```python
from build123d import *

# Parameters (mm, degrees)
SKETCH1_R               = 3.175
SKETCH1_R_2             = 4.025
BOSS_EXTRUDE1_DEPTH     = 6.35
CUT_EXTRUDE2_REACH      = 155.866
CUT_EXTRUDE2_END_RADIUS = 4.025
SKETCH3_R               = 1.1303
FILLET4_R               = 10
SKETCH4_W               = 6.35
SKETCH4_H               = 6.35
SKETCH4_W_2             = 25.4
BOSS_EXTRUDE2_DEPTH     = 4.7625
FILLET3_R               = 2


with BuildPart() as part:
    # Sketch1 → Boss-Extrude1 (new body)
    with BuildSketch(Plane.XY):
        Polygon((-38.1, -12.7), (-38.1, 12.7), (15.701735639, 12.7), (114.28491418, -10.930870684), (108.364133554, -35.631161305), (12.7, -12.7), align=None)
        with Locations((-12.7, 0)):
            Circle(SKETCH1_R, mode=Mode.SUBTRACT)
        with Locations((101.6, -20.95)):
            Circle(SKETCH1_R_2, mode=Mode.SUBTRACT)
    extrude(amount=BOSS_EXTRUDE1_DEPTH)

    # Cut-Extrude2: up to this cylinder (the profile starts outside it)
    cut_extrude2_end = Plane(origin=(101.6, -20.95, 3.175), z_dir=(0, 0, -1)) * Cylinder(CUT_EXTRUDE2_END_RADIUS, 320.782, mode=Mode.PRIVATE)
    # Sketch3 → Cut-Extrude2 (cut, up to the surface)
    with BuildSketch(Plane(origin=(110.552900462, -26.500071647, 0), x_dir=(0, 0, -1), z_dir=(0.9724523866696595, -0.23310159943784806, 0)), mode=Mode.PRIVATE) as cut_extrude2_sk1:
        with Locations(Location((-3.175, 3.310245002, 0), (0, 0, 90))):
            Circle(SKETCH3_R)
    cut_extrude2_tool1 = extrude(cut_extrude2_sk1.sketch, amount=-CUT_EXTRUDE2_REACH, mode=Mode.PRIVATE) - cut_extrude2_end
    add(cut_extrude2_tool1.solids().sort_by_distance((111.324524, -23.281016, 3.175))[0], mode=Mode.SUBTRACT)

    # Fillet4
    fillet4_edges = [part.edges().sort_by_distance(p)[0] for p in [
        (108.364133554, -35.631161305, 3.175),
        (114.28491418, -10.930870684, 3.175),
    ]]
    fillet(fillet4_edges, radius=FILLET4_R)

    # Sketch4 → Boss-Extrude2 (add)
    with BuildSketch(Plane.XY):
        with Locations((-28.575, 0)):
            Rectangle(SKETCH4_W, SKETCH4_H)
        with Locations((7.9375, 0)):
            Rectangle(SKETCH4_W_2, SKETCH4_H)
    extrude(amount=-BOSS_EXTRUDE2_DEPTH)

    # Fillet3
    fillet3_edges = [part.edges().sort_by_distance(p)[0] for p in [
        (12.7, -12.7, 3.175),
        (-38.1, -12.7, 3.175),
        (-38.1, 12.7, 3.175),
        (15.701735639, 12.7, 3.175),
        (-25.4, -3.175, -2.38125),
        (-31.75, -3.175, -2.38125),
        (-31.75, 3.175, -2.38125),
        (-25.4, 3.175, -2.38125),
        (20.6375, -3.175, -2.38125),
        (-4.7625, -3.175, -2.38125),
        (-4.7625, 3.175, -2.38125),
        (20.6375, 3.175, -2.38125),
    ]]
    fillet(fillet3_edges, radius=FILLET3_R)


solid = part.part
```
For this review, take the finished solid that the model builds, in its own axes (mm). A direction names the side the tool comes from. Coordinates: 2 decimals unless noted, no trailing zeros. Loops run counter-clockwise (first coordinate to the right, second up) from the corner with the lowest first, then second, coordinate; pieces in that order, holes last. Notation, with made-up numbers: (16, 42.5) - (44, 42.5) arc R5 cw to (44, 47.5) - close; hole circle Ø3 at (69, 39.25). An arc over 180 degrees is marked (long way). Use one line per item in the form item = value. Start each with the question number.
1) Take a section at A-A (x = -12.7). State the section outline as (y, z) points (3 decimals).
2) Take a section at C-C (x = 101.5). State the section outline as (y, z) points.
3) For faces 4 (the face through (59.63, 2.17, 3.13)), 5 (the face through (8, -3.175, -2)), 6 (the face through (-11, -12.7, 3)), list the 3-axis set-ups (+Z, -Z, +X, -X, +Y, -Y) from which the entire face can be reached by the end or side of a thin tool; tool diameter is ignored.
4) Draft analysis for pull direction Y (two halves, no side actions). For faces 1 (the face through (8, 0, -4.762)), 2 (the face through (-9.67, 0.95, 3.13)), 3 (the face through (8, 3.175, -2)), state which applies: released by +Y, released by -Y, zero draft, split by the parting line, or undercut.
5) Take a section at D-D (y = -27.5). State the section outline as (x, z) points.
6) To check wall thickness, follow probe 1 along Y at (x, z) = (-12.7, 5) (3 decimals); probe 2 along Z at (x, y) = (91, -8); probe 3 along Y at (x, z) = (106, 2.5). State the ranges of each line that lie inside material, in increasing order. Write a range as from..to.
7) For pin 1 (10 mm diameter, centred on x = 20.5, y = -20.5, fed in from -Z); pin 2 (0.7 mm diameter, centred on x = -28, z = -2.5, fed in from -Y) (3 decimals); pin 3 (1 mm diameter, centred on y = -26, z = 3, fed in from +X); pin 4 (5 mm diameter, centred on x = 5, y = -14.5, fed in from -Z), all flat-tipped, find the tip position at first contact; note any pin that passes through.
From the geometry:
q1.outline = (-12.7, 0) - (-3.175, 0) - (-3.175, 6.35) - (-12.7, 6.35) - close; (3.175, 0) - (12.7, 0) - (12.7, 6.35) - (3.175, 6.35) - close
q2.outline = (-33.56, 0) - (-24.97, 0) - (-24.97, 6.35) - (-33.56, 6.35) - close; (-16.93, 0) - (-7.87, 0) - (-7.87, 6.35) - (-16.93, 6.35) - close
q3.face_4 = +Z, -Z, +X, +Y
q3.face_5 = -Z, +X, -X, -Y
q3.face_6 = +Z, -Z, -X, -Y
q4.face_1 = zero draft
q4.face_2 = undercut
q4.face_3 = released by +Y
q5.outline = (74.44, 0) - (110.17, 0) - (110.17, 6.35) - (74.44, 6.35) - close
q6.probe_1 = -12.7..-3.175, 3.175..12.7
q6.probe_2 = 0..6.35
q6.probe_3 = -32.22..-22.94, -21.07..-9.06
q7.pin_1 = through
q7.pin_2 = -3.175
q7.pin_3 = 110.79
q7.pin_4 = 0
